For this review, take the finished solid that the model builds, in its own axes (mm). A direction names the side the tool comes from. Round coordinates to 2 decimals unless told otherwise and drop trailing zeros. Order: outer loops, then holes, each group sorted by start corner. A loop starts at its lowest first (then second) coordinate and runs counter-clockwise, first axis right, second up.
from build123d import *

# Parameters (mm, degrees)
SKETCH1_R           = 76.2
BOSS_EXTRUDE1_DEPTH = 3.81
SKETCH2_R           = 0.7366
CUT_EXTRUDE1_DEPTH  = 108.830404339
CIRPATTERN1_COUNT   = 6
SKETCH3_R           = 6.35
CUT_EXTRUDE2_DEPTH  = 108.830404339
SKETCH5_R           = 3.175
CUT_EXTRUDE3_DEPTH  = 108.830404339
CIRPATTERN2_COUNT   = 8
SKETCH6_W           = 1.27
SKETCH6_H           = 2.54


with BuildPart() as part:
    # Sketch1 → Boss-Extrude1 (new body)
    with BuildSketch(Plane.XY):
        with Locations(Location((0, 0, 0), (0, 0, 180))):
            Circle(SKETCH1_R)
    extrude(amount=BOSS_EXTRUDE1_DEPTH)

    # Sketch2 → Cut-Extrude1 (cut, through all)
    with BuildSketch(Plane(origin=(0, 0, 0), x_dir=(-1, 0, 0), z_dir=(0, 0, -1))):
        with Locations((0, 10.16)):
            Circle(SKETCH2_R)
        with Locations((2.54, 14.559409051)):
            Circle(SKETCH2_R)
        with Locations((5.08, 10.16)):
            Circle(SKETCH2_R)
        with Locations((7.62, 14.559409051)):
            Circle(SKETCH2_R)
        with Locations((-2.54, 14.559409051)):
            Circle(SKETCH2_R)
        with Locations((-5.08, 18.958818102)):
            Circle(SKETCH2_R)
        with Locations((0, 18.958818102)):
            Circle(SKETCH2_R)
        with Locations((5.08, 18.958818102)):
            Circle(SKETCH2_R)
    cut_extrude1 = extrude(amount=-CUT_EXTRUDE1_DEPTH, mode=Mode.SUBTRACT)

    # CirPattern1: Cut-Extrude1 ×6 about axis
    cirpattern1_axis = Axis((0, 0, 0), (0, 0, 1))
    for i in range(1, CIRPATTERN1_COUNT):
        add(cut_extrude1.rotate(cirpattern1_axis, i * 360 / CIRPATTERN1_COUNT), mode=Mode.SUBTRACT)

    # Sketch3 → Cut-Extrude2 (cut, through all)
    with BuildSketch(Plane(origin=(0, 0, 0), x_dir=(-1, 0, 0), z_dir=(0, 0, -1))):
        with Locations((41.275, 0)):
            Circle(SKETCH3_R)
        with Locations((-41.275, 0)):
            Circle(SKETCH3_R)
    extrude(amount=-CUT_EXTRUDE2_DEPTH, mode=Mode.SUBTRACT)

    # Sketch5 → Cut-Extrude3 (cut, through all)
    with BuildSketch(Plane(origin=(0, 0, 0), x_dir=(-1, 0, 0), z_dir=(0, 0, -1))):
        with Locations((66.802, 0)):
            Circle(SKETCH5_R)
    cut_extrude3 = extrude(amount=-CUT_EXTRUDE3_DEPTH, mode=Mode.SUBTRACT)

    # CirPattern2: Cut-Extrude3 ×8 about axis
    cirpattern2_axis = Axis((0, 0, 0), (0, 0, 1))
    for i in range(1, CIRPATTERN2_COUNT):
        add(cut_extrude3.rotate(cirpattern2_axis, i * 360 / CIRPATTERN2_COUNT), mode=Mode.SUBTRACT)

    # Sketch6 → Revolve1 (revolve)
    with BuildSketch(Plane(origin=(0, 0, 0), x_dir=(0, 0, -1), z_dir=(1, 0, 0))):
        with Locations((0.635, 52.07)):
            Rectangle(SKETCH6_W, SKETCH6_H)
    revolve(axis=Axis((0, 0, 0), (0, 0, 1)))


solid = part.part
(1) Wall thickness on L1, parallel to Y at x = -2.54, z = 1.5; L2, parallel to X at y = 44.5, z = 0.3; L3, parallel to X at y = -10.5, z = 0.9: over which ranges is each line inside the solid? List them lowest first.
(2) Add section A-A on x = 28.5. Give the boundary of the cut face in (y, z).
(3) Draft analysis for pull direction X (two halves, no side actions). For faces 1 (the face through (1, -1, 0)), 2 (the face through (16.519, 74.388, 1.878)), 3 (the face through (-47.14, -2.43, 1.88)), 4 (the face through (17, -51, 0)), state which applies: pulls with the +X half, pulls with the -X half, needs draft (parallel to the pull), parting line crosses it, or undercut.
(4) Add section B-B on y = 55.5. Give the boundary of the cut face in (x, z).
(5) Clearance check with flat-ended pins moving along their axes: P1, Ø1.2, axis at x = -11.34, y = 0.68, coming from the -Z side; P2, Ø1.7, axis at x = 5.08, y = -10.16, coming from the -Z side. State where each tip first meets the part, or that it passes through.
(6) Tool access review of faces 5 (the face through (0.14, 63.63, 1.88)), 6 (the face through (49.592, -11.012, -0.644)): name each direction out of +Z, -Z, +X, -X, +Y, -Y from which nothing blocks a thin tool from reaching the whole face with its end or side.
Here are the results:
1. L1: y = -76.16 to -68.71, -64.9 to -15.3, -13.82 to 13.82, 15.3 to 64.9, 68.71 to 76.16
1. L2: x = -61.86 to -48.85, -45.63 to 45.63, 48.85 to 61.86
1. L3: x = -75.47 to -0.65, 0.65 to 4.43, 5.73 to 75.47
2. outline: (-70.67, 0) - (-45.09, 0) - (-45.09, -1.27) - (-42.05, -1.27) - (-42.05, 0) - (42.05, 0) - (42.05, -1.27) - (45.09, -1.27) - (45.09, 0) - (70.67, 0) - (70.67, 3.81) - (-70.67, 3.81) - close
3. face 1: undercut
3. face 2: parting line crosses it
3. face 3: undercut
3. face 4: needs draft
4. outline: (-52.21, 0) - (52.21, 0) - (52.21, 3.81) - (-52.21, 3.81) - close
5. P1: passes through
5. P2: stops at z = 0
6. face 5: +Z, -Z
6. face 6: -Z
